Model file for the job. Use its own axes, mm. A direction names the side the tool comes from. Coordinates: 2 decimals unless noted, no trailing zeros. Write each loop counter-clockwise with the first axis right and the second up, starting at its lowest first coordinate (ties: lowest second). Pieces come first, ordered by that corner, then holes. Notation, with made-up numbers: M -30,58 L 27,58 A5 cw 27,64 Z; hole C -26,-38.75 d11. An arc over 180 degrees is marked long. Put each result on its own line as item: value. Start each with the question number.
Q1. Cut at C-C (x = -3.25). Write the cut outline in (y, z) (3 decimals).
Q2. Cut at B-B (z = 4.25). Write the cut outline in (x, y), then the cut area to 3 significant figures.
Q3. Drop flat-ended pins along their axis: pin 1 (4 mm diameter, centred on y = -9, z = 5.5, fed in from +X); pin 2 (6 mm diameter, centred on x = -7, y = -10, fed in from -Z); pin 3 (6 mm diameter, centred on x = -4, y = -8, fed in from +Z); pin 4 (3 mm diameter, centred on x = 0, y = -1.5, fed in from +Z). Give the stop position or say it passes through.
Q4. Cut at D-D (y = -5.5). Write the cut outline in (x, z).
Q5. Drill centre lines: line 1 along Z through (x, y) = (7.5, -5.5); line 2 along X through (y, z) = (-9, 2); line 3 along X through (y, z) = (-11, -2.25). Where is each one in solid material? Low to high.
Q6. Cut at A-A (y = -8.5). Write the cut outline in (x, z).
Q7. Pull direction X, two halves, no side cores. Call faces 4 (the flat face through (-5, -8, 1.016)), 5 (the flat face through (1.016, -8, -5)): pulls with the +X half, pulls with the -X half, needs draft (parallel to the pull), parting line crosses it, or undercut.
Q8. Which spindle directions (+Z, -Z, +X, -X, +Y, -Y) get a long thin tool onto all of the face, cutting with end or side? Do faces 1 (the flat face through (5, -8, 1.016)), 2 (the flat face through (0, 0, 0)), 3 (the flat face through (1.016, -8, 5)). Say none if no direction does.
```python
from build123d import *

# Parameters (mm, degrees)
F1_ANGLE = 180
F2_W     = 25.4
F2_H     = 2.032
F3_DEPTH = 12.7
F4_W     = 2.032
F4_H     = 25.4
F5_DEPTH = 12.7


with BuildPart() as f1:
    # F0 (on Front) → F1 (revolve)
    with BuildSketch(Plane.XZ):
        with BuildLine():
            ThreePointArc((12.7, 0), (0, 12.7), (-12.7, 0))
            Line((-12.7, 0), (12.7, 0))
        make_face()
    revolve(axis=Axis((0, 0, 0), (1, 0, 0)), revolution_arc=F1_ANGLE)

    # F2 (on Right) → F3 (cut, symmetric)
    with BuildSketch(Plane.YZ):
        with Locations((-17.78, 0)):
            Rectangle(F2_W, F2_H)
    extrude(amount=F3_DEPTH, both=True, mode=Mode.SUBTRACT)

    # F4 (on Top) → F5 (cut, symmetric)
    with BuildSketch(Plane.XY):
        with Locations((0, -17.78)):
            Rectangle(F4_W, F4_H)
    extrude(amount=F5_DEPTH, both=True, mode=Mode.SUBTRACT)


solid = f1.part
```
Computed values:
1. outline: M -12.235,-1.016 A12.277 ccw 0,-12.277 L 0,12.277 A12.277 ccw -12.235,1.016 L -5.08,1.016 L -5.08,-1.016 Z
2. outline: M -11.97,0 A11.97 ccw -1.02,-11.92 L -1.02,-5.08 L 1.02,-5.08 L 1.02,-11.92 A11.97 ccw 11.97,0 Z
2. area: 211 mm2
3. pin 1: x = 9.39
3. pin 2: z = -8.75
3. pin 3: z = 11.22
3. pin 4: z = 12.7
4. outline: M -11.4,-1.02 A11.45 ccw -1.02,-11.4 L -1.02,-1.02 Z; M -11.4,1.02 L -1.02,1.02 L -1.02,11.4 A11.45 ccw Z; M 1.02,-11.4 A11.45 ccw 11.4,-1.02 L 1.02,-1.02 Z; M 1.02,1.02 L 11.4,1.02 A11.45 ccw 1.02,11.4 Z
5. line 1: -8.65 to -1.02, 1.02 to 8.65
5. line 2: -8.73 to -1.02, 1.02 to 8.73
5. line 3: -5.94 to -1.02, 1.02 to 5.94
6. outline: M -9.38,-1.02 A9.44 ccw -1.02,-9.38 L -1.02,-1.02 Z; M -9.38,1.02 L -1.02,1.02 L -1.02,9.38 A9.44 ccw Z; M 1.02,-9.38 A9.44 ccw 9.38,-1.02 L 1.02,-1.02 Z; M 1.02,1.02 L 9.38,1.02 A9.44 ccw 1.02,9.38 Z
7. face 4: needs draft
7. face 5: undercut
8. face 1: +X, -X, -Y
8. face 2: +Z, -Z, +X, -X, +Y
8. face 3: +Z, -Z, -Y
